Read the model definition and answer for the solid it produces. Units are mm, in the model's axes. A direction names the side the tool comes from. Coordinates: 2 decimals unless noted, no trailing zeros. Write each loop counter-clockwise with the first axis right and the second up, starting at its lowest first coordinate (ties: lowest second). Pieces come first, ordered by that corner, then holes. Notation, with made-up numbers: M 88,-8.5 L 117,-8.5 A26 ccw 117,28.5 Z; hole C 49,50 d2. An arc over 180 degrees is marked long. Write item = value, one per line.
from build123d import *

# Parameters (mm, degrees)
SKETCH1_R           = 16.15
SKETCH1_R_2         = 2.4
BOSS_EXTRUDE1_DEPTH = 5


with BuildPart() as part:
    # Sketch1 → Boss-Extrude1 (new body)
    with BuildSketch(Plane.XY):
        with BuildLine():
            Line((12.5, 20), (35, 20))
            Line((35, 20), (35, 0))
            Line((35, 0), (35, -20))
            Line((35, -20), (12.5, -20))
            Line((12.5, -20), (12.5, -63.786754111))
            ThreePointArc((12.5, -63.786754111), (0, -65), (-12.5, -63.786754111))
            Line((-12.5, -63.786754111), (-12.5, -20))
            Line((-12.5, -20), (-35, -20))
            Line((-35, -20), (-35, 20))
            Line((-35, 20), (-12.5, 20))
            Line((-12.5, 20), (-12.5, 63.786754111))
            ThreePointArc((-12.5, 63.786754111), (0, 65), (12.5, 63.786754111))
            Line((12.5, 63.786754111), (12.5, 20))
        make_face()
        Circle(SKETCH1_R, mode=Mode.SUBTRACT)
        with Locations((0, 52)):
            Circle(SKETCH1_R_2, mode=Mode.SUBTRACT)
        with Locations((30, 0)):
            Circle(SKETCH1_R_2, mode=Mode.SUBTRACT)
        with Locations((0, -52)):
            Circle(SKETCH1_R_2, mode=Mode.SUBTRACT)
        with Locations((-30, 0)):
            Circle(SKETCH1_R_2, mode=Mode.SUBTRACT)
    extrude(amount=BOSS_EXTRUDE1_DEPTH)


solid = part.part
Item 1: Find section C-C (x = 0). Determine the outline of the cut face in (y, z), and give its area (4 significant figures).
Worked answers:
outline = M -65,0 L -54.4,0 L -54.4,5 L -65,5 Z; M -49.6,0 L -16.15,0 L -16.15,5 L -49.6,5 Z; M 16.15,0 L 49.6,0 L 49.6,5 L 16.15,5 Z; M 54.4,0 L 65,0 L 65,5 L 54.4,5 Z
area = 440.5 mm²
Item 2: Which of the six approach directions +Z, -Z, +X, -X, +Y, -Y give full straight-line access (tool end or side, diameter ignored) to faces 1 (the face through (24, 20, 2)), 2 (the face through (24, -20, 2)), 3 (the face through (-24, -20, 2))?
Worked answers:
face_1 = +Z, -Z, +X, +Y
face_2 = +Z, -Z, +X, -Y
face_3 = +Z, -Z, -X, -Y
Item 3: For a pull along X with two mould halves and no side action, classify faces 4 (the face through (8, 15, 5)), 5 (the face through (-12.5, 42, 2)), 6 (the face through (0, 65, 2)), 7 (the face through (1.11, -54.13, 2.46)) as released by +X, released by -X, zero draft, split by the parting line, or undercut.
Worked answers:
face_4 = zero draft
face_5 = released by -X
face_6 = split by the parting line
face_7 = undercut
Item 4: Find section B-B (y = 52). Determine the outline of the cut face in (x, z), and give its area (3 significant figures).
Worked answers:
outline = M -12.5,0 L -2.4,0 L -2.4,5 L -12.5,5 Z; M 2.4,0 L 12.5,0 L 12.5,5 L 2.4,5 Z
area = 101 mm²
Item 5: Flat-ended cylindrical pins translate along their axes: pin 1 (1.5 mm diameter, centred on x = 21.5, z = 2, fed in from -Y); pin 2 (1.5 mm diameter, centred on y = 46, z = 2.5, fed in from -X); pin 3 (2.5 mm diameter, centred on y = -42, z = 2, fed in from +X). Find the tip coordinate at first contact, or state that the pin passes through.
Worked answers:
pin_1 = -20
pin_2 = -12.5
pin_3 = 12.5
Item 6: Find section D-D (y = 0). Determine the outline of the cut face in (x, z).
Worked answers:
outline = M -35,0 L -32.4,0 L -32.4,5 L -35,5 Z; M -27.6,0 L -16.15,0 L -16.15,5 L -27.6,5 Z; M 16.15,0 L 27.6,0 L 27.6,5 L 16.15,5 Z; M 32.4,0 L 35,0 L 35,5 L 32.4,5 Z
Item 7: Consider line 1 along Y through (x, z) = (0, 3.9); line 2 along Y through (x, z) = (-30, 1.05); line 3 along X through (y, z) = (27.5, 2.9). Determine where each line is inside the solid, lowest interval first. Write a range as from..to.
Worked answers:
line_1 = -65..-54.4, -49.6..-16.15, 16.15..49.6, 54.4..65
line_2 = -20..-2.4, 2.4..20
line_3 = -12.5..12.5
Item 8: Find section A-A (x = -30). Determine the outline of the cut face in (y, z), and give its area (3 significant figures).
Worked answers:
outline = M -20,0 L -2.4,0 L -2.4,5 L -20,5 Z; M 2.4,0 L 20,0 L 20,5 L 2.4,5 Z
area = 176 mm²
